Answer from the drawing. Dimensions are ordinates in mm from the lowest x, y and z of the part. Coordinates: 2 decimals unless noted, no trailing zeros. Write each loop counter-clockwise with the first axis right and the second up, starting at its lowest first coordinate (ties: lowest second). Pieces come first, ordered by that corner, then holes.
(1) The part is cut by section A-A, the plane y = 1.7. Determine the outline of the cut face in (x, z), and give its area (3 significant figures).
(2) The part is cut by section B-B, the plane z = 32.5. Determine the outline of the cut face in (x, y), and give its area (3 significant figures).
(3) The part is cut by section C-C, the plane x = 32.5. Determine the outline of the cut face in (y, z).
(4) Straight lines are drawn through the part: line 1 along Z through (x, y) = (31.5, 1.25); line 2 along X through (y, z) = (2.85, 6). For each, find the intervals that lie inside material, in ascending order.
(5) Given pin 1 (0.9 mm diameter, centred on x = 4.5, y = 2, fed in from -Z); pin 2 (1.5 mm diameter, centred on y = 2, z = 59.5, fed in from -X); pin 3 (0.9 mm diameter, centred on y = 1.5, z = 32, fed in from -X), each flat-ended and moving along its own axis, determine where each tip first touches the part or whether it passes through.
(6) The part is cut by section D-D, the plane x = 10.5. Determine the outline of the cut face in (y, z), and give its area (3 significant figures).
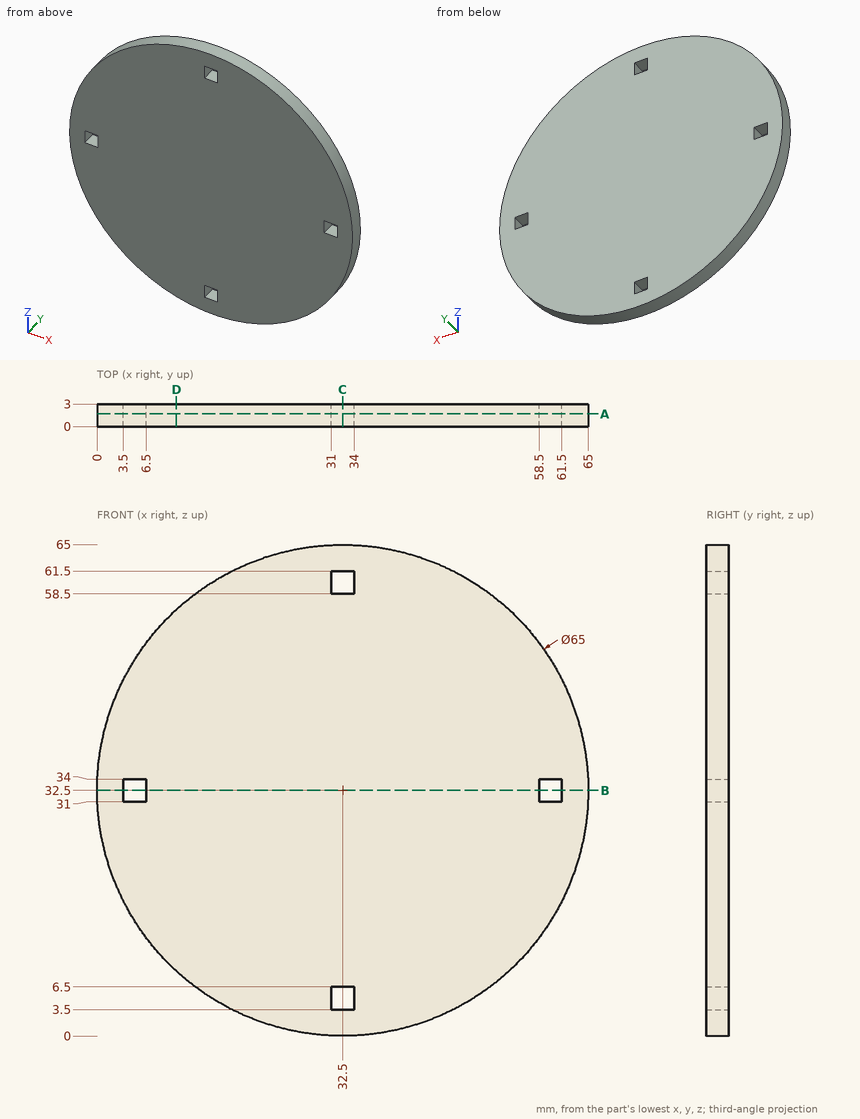
Computed:
1. outline: circle Ø65 at (32.5, 32.5); hole (3.5, 31) - (6.5, 31) - (6.5, 34) - (3.5, 34) - close; hole (31, 3.5) - (34, 3.5) - (34, 6.5) - (31, 6.5) - close; hole (31, 58.5) - (34, 58.5) - (34, 61.5) - (31, 61.5) - close; hole (58.5, 31) - (61.5, 31) - (61.5, 34) - (58.5, 34) - close
1. area: 3,280 mm2
2. outline: (0, 0) - (3.5, 0) - (3.5, 3) - (0, 3) - close; (6.5, 0) - (58.5, 0) - (58.5, 3) - (6.5, 3) - close; (61.5, 0) - (65, 0) - (65, 3) - (61.5, 3) - close
2. area: 177 mm2
3. outline: (0, 0) - (3, 0) - (3, 3.5) - (0, 3.5) - close; (0, 6.5) - (3, 6.5) - (3, 58.5) - (0, 58.5) - close; (0, 61.5) - (3, 61.5) - (3, 65) - (0, 65) - close
4. line 1: z = 0.02 to 3.5, 6.5 to 58.5, 61.5 to 64.98
4. line 2: x = 13.69 to 31, 34 to 51.31
5. pin 1: stops at z = 15.26
5. pin 2: stops at x = 13.34
5. pin 3: stops at x = 0
6. outline: (0, 8.58) - (3, 8.58) - (3, 56.42) - (0, 56.42) - close
6. area: 144 mm2
